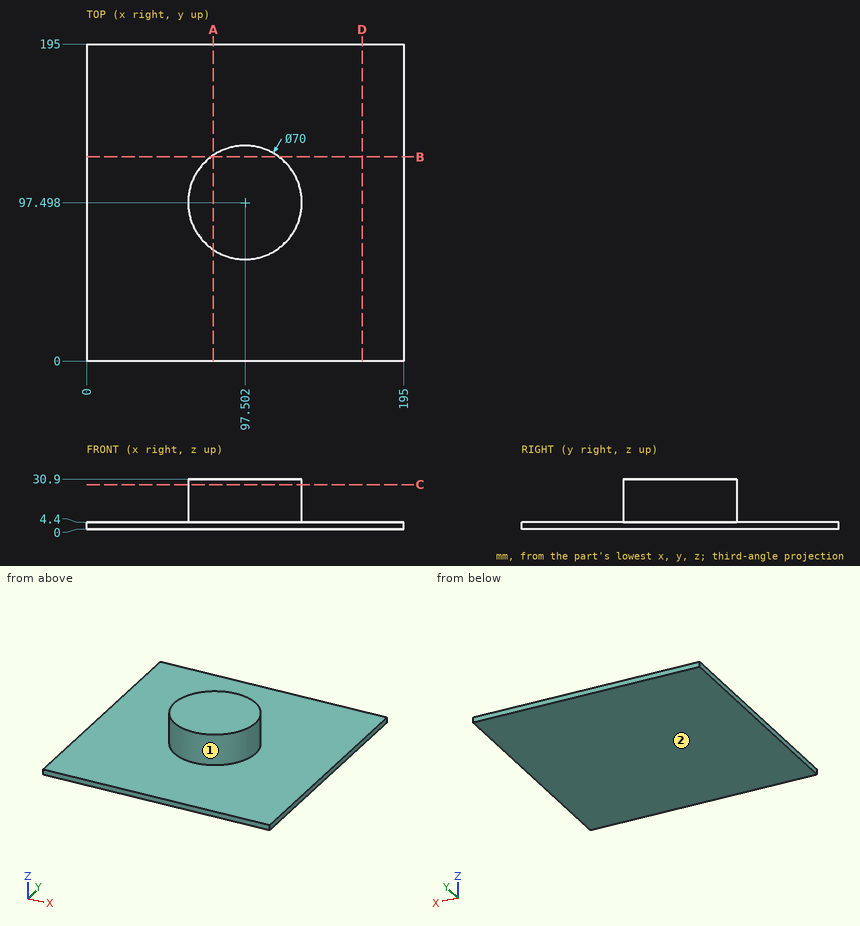
The drawing under review shows one solid part. Ordinate dimensions are in mm from its lowest x, y, z. A direction names the side the tool comes from. Round coordinates to 2 decimals unless told otherwise and drop trailing zeros. Loops run counter-clockwise (first coordinate to the right, second up) from the corner with the lowest first, then second, coordinate; pieces in that order, holes last.
Item 1: Take a section at D-D (x = 169.5). Write out the cut boundary in (y, z).
Determined:
outline: (0, 0) - (195, 0) - (195, 4.4) - (0, 4.4) - close
Item 2: For the marked faces 1 and 2, list the 3-axis set-ups (+Z, -Z, +X, -X, +Y, -Y) from which the entire face can be reached by the end or side of a thin tool; tool diameter is ignored.
Determined:
face 1: +Z
face 2: -Z, +X, -X, +Y, -Y
Item 3: Take a section at C-C (z = 27.5). Write out the cut boundary in (x, y), then the cut area to 3 significant figures.
Determined:
outline: circle Ø70 at (97.5, 97.5)
area: 3,850 mm2
Item 4: Take a section at A-A (x = 78). Write out the cut boundary in (y, z).
Determined:
outline: (0, 0) - (195, 0) - (195, 4.4) - (126.56, 4.4) - (126.56, 30.9) - (68.43, 30.9) - (68.43, 4.4) - (0, 4.4) - close
Item 5: For line 1 (Z direction, x = 178.5, y = 98); line 2 (Y direction, x = 75, z = 13); line 3 (X direction, y = 103, z = 28), list the stretches that pass through material, from the lowest coordinate up.
Determined:
line 1: z = 0 to 4.4
line 2: y = 70.69 to 124.31
line 3: x = 62.94 to 132.07
Item 6: Take a section at B-B (y = 125.5). Write out the cut boundary in (x, z) (1 decimal), then the cut area to 3 significant figures.
Determined:
outline: (0, 0) - (195, 0) - (195, 4.4) - (118.5, 4.4) - (118.5, 30.9) - (76.5, 30.9) - (76.5, 4.4) - (0, 4.4) - close
area: 1,970 mm2
Item 7: Clearance check with flat-ended pins moving along their axes: pin 1 Ø4 at (y, z) = (125, 8.5) entering from +X; pin 2 Ø2 at (x, z) = (126, 26) entering from -Y (1 decimal). State where each tip first meets the part, or that it passes through.
Determined:
pin 1: stops at x = 121.47
pin 2: stops at y = 75.8
